Build history of the part. All positions in model axes, mm. A direction names the side the tool comes from. Give positions to 0.01 mm unless a question says otherwise; leave off trailing zeros. Loops run counter-clockwise (first coordinate to the right, second up) from the corner with the lowest first, then second, coordinate; pieces in that order, holes last. Notation, with made-up numbers: (27, 41.25) - (56, 41.25) arc R21 ccw to (56, 65.25) - close; hole circle Ø2 at (0.5, 84.5). An arc over 180 degrees is marked (long way). Return JSON: item names as keys, results as strings. Group by question number.
1) Slice it at B-B (z = 0). List the corners of the cut face in (x, y).
2) Drop flat-ended pins along their axis: pin 1 (5 mm diameter, centred on x = 13.5, z = 27.5, fed in from -Y); pin 2 (4 mm diameter, centred on x = 12.5, z = 8.5, fed in from -Y); pin 3 (12 mm diameter, centred on y = -13, z = -26, fed in from +X); pin 4 (12 mm diameter, centred on y = -16.5, z = -1.5, fed in from -X). Give the stop position or say it passes through.
3) Drill centre lines: probe 1 along X at (y, z) = (-2, 0); probe 2 along X at (y, z) = (-16.5, 0); probe 3 along X at (y, z) = (-4.5, 8.5). Where is each one in solid material? Low to high. Write a range as from..to.
4) Slice it at C-C (x = 0). List the corners of the cut face in (y, z), and give its area (3 significant figures).
5) Slice it at A-A (y = 0). List the corners of the cut face in (x, z), and give its area (3 significant figures).
6) 3-axis set-ups, long thin cutter, end or side, ignore diameter. For faces 4 (the face through (19.3, -24.91, -12.31)), 5 (the face through (-1, 5, -22)): which of +Z, -Z, +X, -X, +Y, -Y reach the whole face in a straight line?
7) Slice it at D-D (y = -37). List the corners of the cut face in (x, z).
8) Mould opens along Z. For faces 1 (the face through (-16.274, -21.039, -8.465)), 2 (the face through (19, -45.386, 0)), 3 (the face through (-97.495, 0.07, -0.495)) say: released by +Z, released by -Z, zero draft, split by the parting line, or undercut.
```python
from build123d import *

# Parameters (mm, degrees)
SKETCH1_R           = 17.785523023
SKETCH1_R_2         = 10
BOSS_EXTRUDE1_DEPTH = 5
SKETCH2_R           = 22.889678729
BOSS_EXTRUDE2_DEPTH = 40.386280802
SKETCH4_R           = 18.343761553
CUT_EXTRUDE1_DEPTH  = 60
FILLET1_R           = 1


with BuildPart() as part:
    # Sketch1 → Boss-Extrude1 (new, symmetric)
    with BuildSketch(Plane(origin=(0, 0, 0), x_dir=(1, 0, 0), z_dir=(0, 1, 0))):
        with BuildLine():
            Line((-75, -22.5), (-3.19997264, -36.813396757))
            ThreePointArc((-3.19997264, -36.813396757), (0.426652195, -37.154633481), (4.043342361, -36.720579984))
            Line((4.043342361, -36.720579984), (74.823113208, -22.5))
            ThreePointArc((74.823113208, -22.5), (97.323113208, 0), (74.823113208, 22.5))
            Line((74.823113208, 22.5), (3.537735849, 42.902368838))
            ThreePointArc((3.537735849, 42.902368838), (-0.088443396, 43.290961135), (-3.714622642, 42.902368838))
            Line((-3.714622642, 42.902368838), (-75, 22.5))
            ThreePointArc((-75, 22.5), (-97.5, 0), (-75, -22.5))
        make_face()
        with Locations(Location((0, 0, 0), (0, 0, 270))):
            Circle(SKETCH1_R, mode=Mode.SUBTRACT)
        with Locations(Location((-75, 0, 0), (0, 0, 270))):
            Circle(SKETCH1_R_2, mode=Mode.SUBTRACT)
        with Locations(Location((74.823113208, 0, 0), (0, 0, 90))):
            Circle(SKETCH1_R_2, mode=Mode.SUBTRACT)
    extrude(amount=BOSS_EXTRUDE1_DEPTH, both=True)

    # Sketch2 → Boss-Extrude2 (add)
    with BuildSketch(Plane.XZ.offset(5)):
        with Locations(Location((0, 0, 0), (0, 0, 270))):
            Circle(SKETCH2_R)
    extrude(amount=BOSS_EXTRUDE2_DEPTH)

    # Sketch4 → Cut-Extrude1 (cut)
    with BuildSketch(Plane.XZ.offset(45.386280802)):
        with Locations(Location((0, 0, 0), (0, 0, 270))):
            Circle(SKETCH4_R)
    extrude(amount=-CUT_EXTRUDE1_DEPTH, mode=Mode.SUBTRACT)

    # Fillet1
    fillet1_edges = [part.edges().sort_by_distance(p)[0] for p in [
        (0, 5, 18.343761553),
    ]]
    fillet(fillet1_edges, radius=FILLET1_R)


solid = part.part
```
Results:
{
 "1": {"outline": "(-97.5, -5) - (-85, -5) - (-85, 5) - (-97.5, 5) - close; (-65, -5) - (-22.89, -5) - (-22.89, -45.39) - (-18.34, -45.39) - (-18.34, 4) arc R1 ccw to (-19.34, 5) - (-65, 5) - close; (18.34, -45.39) - (22.89, -45.39) - (22.89, -5) - (64.82, -5) - (64.82, 5) - (19.34, 5) arc R1 ccw to (18.34, 4) - close; (84.82, -5) - (97.32, -5) - (97.32, 5) - (84.82, 5) - close"},
 "2": {"pin 1": "y = -5", "pin 2": "through", "pin 3": "x = 11.13", "pin 4": "x = -22.89"},
 "3": {"probe 1": "-97.5..-85, -65..-18.34, 18.34..64.82, 84.82..97.32", "probe 2": "-22.89..-18.34, 18.34..22.89", "probe 3": "-95.83..-80.27, -69.73..-16.26, 16.26..69.56, 80.09..95.66"},
 "4": {"outline": "(-45.39, -22.89) - (-5, -22.89) - (-5, -43.29) - (5, -43.29) - (5, -19.34) arc R1 ccw to (4, -18.34) - (-45.39, -18.34) - close; (-45.39, 18.34) - (4, 18.34) arc R1 ccw to (5, 19.34) - (5, 37.15) - (-5, 37.15) - (-5, 22.89) - (-45.39, 22.89) - close", "area": "804 mm2"},
 "5": {"outline": "(-75, -22.5) - (-3.71, -42.9) arc R17.11 ccw to (3.54, -42.9) - (74.82, -22.5) arc R22.5 ccw to (74.82, 22.5) - (4.04, 36.72) arc R17.11 ccw to (-3.2, 36.81) - (-75, 22.5) arc R22.5 ccw to start; hole circle Ø20 at (-75, 0); hole circle Ø36.69 at (0, 0); hole circle Ø20 at (74.82, 0)", "area": "9,370 mm2"},
 "6": {"face 4": "-Y", "face 5": "+Z, -Z, +X, -X, +Y"},
 "7": {"outline": "circle Ø45.78 at (0, 0); hole circle Ø36.69 at (0, 0)"},
 "8": {"face 1": "undercut", "face 2": "zero draft", "face 3": "split by the parting line"}
}
